```python
from build123d import *

# Parameters (mm, degrees)
F0_R     = 25
F1_DEPTH = 50
F2_R     = 4.5
F3_R     = 15
F4_DEPTH = 6
F5_D     = 3.3
F5_DEPTH = 8
F5_TIP   = 0.9914200214
F6_R     = 4
F7_DEPTH = 17


with BuildPart() as f1:
    # F0 (on Front) → F1 (new body)
    with BuildSketch(Plane.XZ):
        Circle(F0_R)
    extrude(amount=-F1_DEPTH)

    # F2
    f2_edges = [f1.edges().sort_by_distance(p)[0] for p in [
        (-25, 50, 0),
    ]]
    fillet(f2_edges, radius=F2_R)

    # F3 (on face) → F4 (join)
    with BuildSketch(Plane.XZ):
        Circle(F3_R)
    extrude(amount=F4_DEPTH)

    # F5
    with Locations(Plane.XZ):
        with Locations((0, 19), (-16.4544826719, -9.5), (16.4544826719, -9.5)):
            Hole(F5_D / 2, depth=F5_DEPTH)
            with Locations((0, 0, -(F5_DEPTH + F5_TIP / 2))):  # 118° drill point
                Cone(0, F5_D / 2, F5_TIP, mode=Mode.SUBTRACT)

    # F6 (on face) → F7 (join)
    with BuildSketch(Plane.XZ.offset(6)):
        Circle(F6_R)
    extrude(amount=F7_DEPTH)


solid = f1.part
```
Model file for the job. Use its own axes, mm. A direction names the side the tool comes from. Coordinates: 2 decimals unless noted, no trailing zeros. Write each loop counter-clockwise with the first axis right and the second up, starting at its lowest first coordinate (ties: lowest second). Pieces come first, ordered by that corner, then holes. Notation, with made-up numbers: (-29, 67.5) - (23, 67.5) arc R17 cw to (23, 77.5) - close; hole circle Ø2 at (48, 26.5). An arc over 180 degrees is marked (long way). Use a Markdown table: item, result. Add a question column.
Item 1: Band-saw the part on C-C, the plane y = -4.5. Write the cut outline in (x, z).
Item 2: Band-saw the part on D-D, the plane y = 39. Write the cut outline in (x, z), and give its area (3 significant figures).
Item 3: Drop flat-ended pins along their axis: pin 1 (2.5 mm diameter, centred on x = 0, z = 19, fed in from -Y); pin 2 (3 mm diameter, centred on x = 2, y = -14, fed in from +Z); pin 3 (5 mm diameter, centred on y = 5, z = 1.5, fed in from +X); pin 4 (12 mm diameter, centred on y = 29, z = -10.5, fed in from -X). Give the stop position or say it passes through.
Item 4: Band-saw the part on B-B, the plane z = 0. Write the cut outline in (x, y).
Item 5: Band-saw the part on A-A, the plane y = 5. Write the cut outline in (x, z).
Item 6: 3-axis set-ups, long thin cutter, end or side, ignore diameter. For faces 4 (the face through (0.215, 4.056, 20.636)), 5 (the face through (0, -23, 0)): which of +Z, -Z, +X, -X, +Y, -Y reach the whole face in a straight line?
Item 7: Two-plate mould, pull along Z, no slides. Class faces 1 (the face through (-17.98, 4.06, -10.13)), 2 (the face through (-14.985, -2.958, 0.66)), 3 (the face through (0, 50, 0)): pulls with the +Z half, pulls with the -Z half, needs draft (parallel to the pull), parting line crosses it, or undercut.
Item 8: Drill centre lines: line 1 along Z through (x, y) = (0, 3.25); line 2 along X through (y, z) = (6.25, -9.5); line 3 along X through (y, z) = (36, -20). Where is each one in solid material? Low to high.
A:
| question | item | result |
|---|---|---|
| 1 | outline | circle Ø30 at (0, 0) |
| 2 | outline | circle Ø50 at (0, 0) |
| 2 | area | 1,960 mm² |
| 3 | pin 1 | stops at y = 8.24 |
| 3 | pin 2 | stops at z = 3.97 |
| 3 | pin 3 | stops at x = 25 |
| 3 | pin 4 | stops at x = -24.59 |
| 4 | outline | (-25, 0) - (-15, 0) - (-15, -6) - (-4, -6) - (-4, -23) - (4, -23) - (4, -6) - (15, -6) - (15, 0) - (25, 0) - (25, 45.5) arc R4.5 ccw to (20.5, 50) - (-20.5, 50) arc R4.5 ccw to (-25, 45.5) - close |
| 5 | outline | circle Ø50 at (0, 0); hole circle Ø3.3 at (-16.45, -9.5); hole circle Ø3.3 at (0, 19); hole circle Ø3.3 at (16.45, -9.5) |
| 6 | face 4 | -Y |
| 6 | face 5 | +Z, -Z, +X, -X, -Y |
| 7 | face 1 | undercut |
| 7 | face 2 | parting line crosses it |
| 7 | face 3 | needs draft |
| 8 | line 1 | z = -25 to 17.35, 20.65 to 25 |
| 8 | line 2 | x = -23.12 to -18.1, -14.8 to 14.8, 18.1 to 23.12 |
| 8 | line 3 | x = -15 to 15 |
